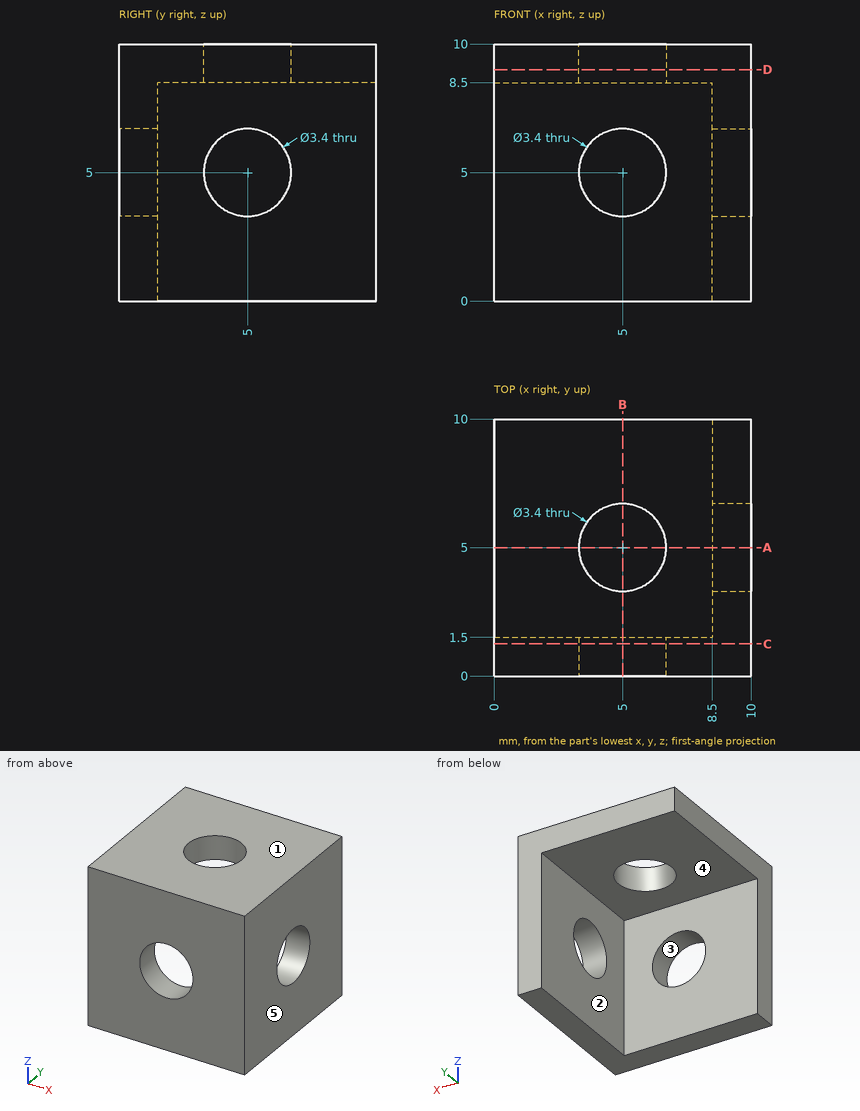
Answer from the drawing. Dimensions are ordinates in mm from the lowest x, y and z of the part. A direction names the side the tool comes from. Round coordinates to 2 decimals unless told otherwise and drop trailing zeros. Write each loop counter-clockwise with the first axis right and the second up, starting at its lowest first coordinate (ties: lowest second). Pieces come first, ordered by that corner, then holes. Notation, with made-up numbers: (8, -13.5) - (44, -13.5) arc R10 ccw to (44, -9.5) - close; hole circle Ø9 at (88, 30.5). An arc over 180 degrees is marked (long way). Use a Markdown table: item, result.
(1) Straight lines are drawn through the part: line 1 along Y through (x, z) = (5, 9.05); line 2 along X through (y, z) = (7.5, 5). For each, find the intervals that lie inside material, in ascending order. Write a range as [from, to].
Reported:
| item | result |
|---|---|
| line 1 | [0, 3.3], [6.7, 10] |
| line 2 | [8.5, 10] |
(2) The part is cut by section A-A (y = 5). Write down the section's boundary in (x, z).
Reported:
| item | result |
|---|---|
| outline | (0, 8.5) - (3.3, 8.5) - (3.3, 10) - (0, 10) - close; (6.7, 8.5) - (8.5, 8.5) - (8.5, 6.7) - (10, 6.7) - (10, 10) - (6.7, 10) - close; (8.5, 0) - (10, 0) - (10, 3.3) - (8.5, 3.3) - close |
(3) The mould has two halves that part along X. Classify the marked faces 3, 4 and 5: released by +X, released by -X, zero draft, split by the parting line, or undercut.
Reported:
| item | result |
|---|---|
| face 3 | undercut |
| face 4 | zero draft |
| face 5 | released by +X |
(4) Which of the six approach directions +Z, -Z, +X, -X, +Y, -Y give full straight-line access (tool end or side, diameter ignored) to the marked faces 1 and 2?
Reported:
| item | result |
|---|---|
| face 1 | +Z, +X, -X, +Y, -Y |
| face 2 | -Z, -X, +Y |
(5) The part is cut by section C-C (y = 1.25). Write down the section's boundary in (x, z), then the cut area to 3 significant figures.
Reported:
| item | result |
|---|---|
| outline | (0, 0) - (10, 0) - (10, 10) - (0, 10) - close; hole circle Ø3.4 at (5, 5) |
| area | 90.9 mm2 |
(6) The part is cut by section B-B (x = 5). Write down the section's boundary in (y, z), then the cut area to 4 significant figures.
Reported:
| item | result |
|---|---|
| outline | (0, 0) - (1.5, 0) - (1.5, 3.3) - (0, 3.3) - close; (0, 6.7) - (1.5, 6.7) - (1.5, 8.5) - (3.3, 8.5) - (3.3, 10) - (0, 10) - close; (6.7, 8.5) - (10, 8.5) - (10, 10) - (6.7, 10) - close |
| area | 17.55 mm2 |
(7) Each of these flat-tipped pins is pushed along its axis until it touches: pin 1 Ø4 at (y, z) = (5.5, 5.5) entering from -X; pin 2 Ø4 at (x, y) = (2, 6.5) entering from -Z; pin 3 Ø4 at (x, z) = (5.5, 5.5) entering from +Y. Where does it stop, or does it pass through?
Reported:
| item | result |
|---|---|
| pin 1 | x = 8.5 |
| pin 2 | z = 8.5 |
| pin 3 | y = 1.5 |
